Work out the finished part from the listing and answer in its coordinate system (mm). Give positions to 0.01 mm unless a question says otherwise; leave off trailing zeros. Order: outer loops, then holes, each group sorted by start corner. A loop starts at its lowest first (then second) coordinate and runs counter-clockwise, first axis right, second up. Notation, with made-up numbers: M -14,40.5 L 33,40.5 A27 cw 33,75.5 Z; hole C 88.25,28 d3. An arc over 180 degrees is marked long. One line per item, written item: value.
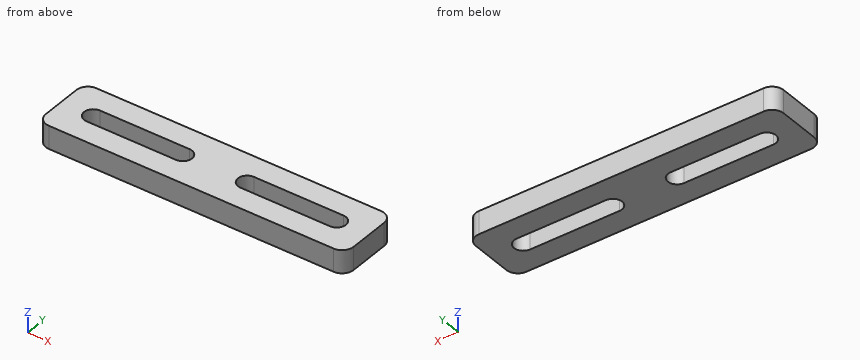
from build123d import *

# Parameters (mm, degrees)
F1_DEPTH = 10
F2_R     = 5


with BuildPart() as f1:
    # F0 (on Top) → F1 (new body)
    with BuildSketch(Plane.XY):
        Polygon((53, 14), (-14, 14), (-14, -14), (53, -14), (120, -14), (120, 14), align=None)
        with BuildLine():
            ThreePointArc((0, -4), (-4, 0), (0, 4))
            Line((0, 4), (39, 4))
            ThreePointArc((39, 4), (43, 0), (39, -4))
            Line((39, -4), (0, -4))
        make_face(mode=Mode.SUBTRACT)
        with BuildLine():
            Line((67, 4), (106, 4))
            ThreePointArc((106, 4), (110, 0), (106, -4))
            Line((106, -4), (67, -4))
            ThreePointArc((67, -4), (63, 0), (67, 4))
        make_face(mode=Mode.SUBTRACT)
    extrude(amount=F1_DEPTH)

    # F2
    f2_edges = [f1.edges().sort_by_distance(p)[0] for p in [
        (-14, 14, 5),
        (-14, -14, 5),
        (120, -14, 5),
        (120, 14, 5),
    ]]
    fillet(f2_edges, radius=F2_R)


solid = f1.part
(1) Find the intervals of material crossed by probe 1 along Y at (x, z) = (80, 3.5); probe 2 along X at (y, z) = (-3.5, 1.75); probe 3 along Y at (x, z) = (107.5, 9.75), in increasing order. Write a range as from..to.
Findings:
probe 1: y = -14..-4, 4..14
probe 2: x = -14..-1.94, 40.94..65.06, 107.94..120
probe 3: y = -14..-3.71, 3.71..14
(2) Section B-B, the plane z = 2.5 is taken. Give the vertices of the cut face in (x, y).
Findings:
outline: M -14,-9 A5 ccw -9,-14 L 115,-14 A5 ccw 120,-9 L 120,9 A5 ccw 115,14 L -9,14 A5 ccw -14,9 Z; hole M 0,-4 L 39,-4 A4 ccw 39,4 L 0,4 A4 ccw Z; hole M 67,-4 L 106,-4 A4 ccw 106,4 L 67,4 A4 ccw Z
(3) Given P1, Ø4, axis at y = 10, z = 2.5, coming from the -X side; P2, Ø3, axis at x = 74, y = 2, coming from the -Z side, each flat-ended and moving along its own axis, determine where each tip first touches the part or whether it passes through.
Findings:
P1: stops at x = -14
P2: passes through
(4) Section A-A, the plane x = 104.5 is taken. Give the vertices of the cut face in (y, z), then the cut area to 3 significant figures.
Findings:
outline: M -14,0 L -4,0 L -4,10 L -14,10 Z; M 4,0 L 14,0 L 14,10 L 4,10 Z
area: 200 mm^2
(5) Section C-C, the plane y = 0 is taken. Give the vertices of the cut face in (x, z).
Findings:
outline: M -14,0 L -4,0 L -4,10 L -14,10 Z; M 43,0 L 63,0 L 63,10 L 43,10 Z; M 110,0 L 120,0 L 120,10 L 110,10 Z
